Part model, mm, in its own coordinate system. A direction names the side the tool comes from. Give positions to 0.01 mm unless a question says otherwise; leave off trailing zeros. Write each loop counter-clockwise with the first axis right and the second up, starting at its lowest first coordinate (ties: lowest second). Pieces come first, ordered by that corner, then holes. Notation, with made-up numbers: (58.25, 43.5) - (63.25, 43.5) arc R28 cw to (63.25, 68.5) - close; hole circle Ø8 at (39.25, -2). An arc over 180 degrees is marked (long way). Answer in a Markdown table with one row per item. Add a question column.
1. Pull direction Y, two halves, no side cores. Call faces 6 (the flat face through (9, 20.857, 1)), 7 (the flat face through (9, 1, 11.429)), 8 (the flat face through (9, 0, 6)), 9 (the cylindrical face through (8.064, 18.249, 4.972)): released by +Y, released by -Y, zero draft, split by the parting line, or undercut.
2. Which spindle directions (+Z, -Z, +X, -X, +Y, -Y) get a long thin tool onto all of the face, cutting with end or side? Do faces 1 (the flat face through (17.714, 1, 6)), 2 (the flat face through (9, 7, 0)), 3 (the flat face through (9, 19, 7)), 4 (the flat face through (7.357, 11, 1)), 5 (the flat face through (10.357, 11, 1)). Say none if no direction does.
3. Drop flat-ended pins along their axis: pin 1 Ø2 at (y, z) = (10, 1.5) entering from -X; pin 2 Ø3 at (x, z) = (6, 4.5) entering from +Y; pin 3 Ø0.6 at (x, y) = (8.5, 19) entering from +Z. Give the stop position or say it passes through.
4. Probe line 1 along Y through (x, z) = (11, 5.25); line 2 along X through (y, z) = (18.75, 5.5); line 3 along X through (y, z) = (15.75, 1.75). List the from-to ranges inside material, lowest first.
5. Band-saw the part on B-B on z = 1.5. Write the cut outline in (x, y), plus the area to 3 significant figures.
6. Band-saw the part on D-D on y = 15. Write the cut outline in (x, z).
7. Band-saw the part on A-A on z = 4.5. Write the cut outline in (x, y).
8. Band-saw the part on C-C on x = 9.5. Write the cut outline in (y, z).
```python
from build123d import *

# Parameters (mm, degrees)
F1_W     = 3
F1_H     = 18.8571428571
F1_R     = 1
F2_DEPTH = 3
F3_DEPTH = 11.4285714286
F4_DEPTH = 7


with BuildPart() as f2:
    # F1 (on Top) → F2 (new body)
    with BuildSketch(Plane.XY):
        with Locations((8.8571428571, 11.4285714286)):
            Rectangle(F1_W, F1_H)
        with Locations((8.8571428571, 18.8571428571)):
            Circle(F1_R, mode=Mode.SUBTRACT)
        Polygon((0, 2), (0, 0), (17.7142857143, 0), (17.7142857143, 2), (10.3571428571, 2), (7.3571428571, 2), align=None)
        with Locations((8.8571428571, 18.8571428571)):
            Circle(F1_R)
    extrude(amount=F2_DEPTH)

    # F1 (on Top) → F3 (join)
    with BuildSketch(Plane.XY):
        Polygon((0, 2), (0, 0), (17.7142857143, 0), (17.7142857143, 2), (10.3571428571, 2), (7.3571428571, 2), align=None)
    extrude(amount=F3_DEPTH)

    # F1 (on Top) → F4 (join)
    with BuildSketch(Plane.XY):
        with Locations((8.8571428571, 18.8571428571)):
            Circle(F1_R)
    extrude(amount=F4_DEPTH)


solid = f2.part
```
Values:
| question | item | result |
|---|---|---|
| 1 | face 6 | released by +Y |
| 1 | face 7 | zero draft |
| 1 | face 8 | released by -Y |
| 1 | face 9 | undercut |
| 2 | face 1 | +Z, -Z, +X, +Y, -Y |
| 2 | face 2 | -Z, +X, -X, +Y, -Y |
| 2 | face 3 | +Z, +X, -X, +Y |
| 2 | face 4 | +Z, -Z, -X, +Y |
| 2 | face 5 | +Z, -Z, +X, +Y |
| 3 | pin 1 | stops at x = 7.36 |
| 3 | pin 2 | stops at y = 2 |
| 3 | pin 3 | stops at z = 7 |
| 4 | line 1 | y = 0 to 2 |
| 4 | line 2 | x = 7.86 to 9.85 |
| 4 | line 3 | x = 7.36 to 10.36 |
| 5 | outline | (0, 0) - (17.71, 0) - (17.71, 2) - (10.36, 2) - (10.36, 20.86) - (7.36, 20.86) - (7.36, 2) - (0, 2) - close |
| 5 | area | 92.0 mm² |
| 6 | outline | (7.36, 0) - (10.36, 0) - (10.36, 3) - (7.36, 3) - close |
| 7 | outline | (0, 0) - (17.71, 0) - (17.71, 2) - (0, 2) - close; circle Ø2 at (8.86, 18.86) |
| 8 | outline | (0, 0) - (20.86, 0) - (20.86, 3) - (19.62, 3) - (19.62, 7) - (18.09, 7) - (18.09, 3) - (2, 3) - (2, 11.43) - (0, 11.43) - close |
